from build123d import *

# Parameters (mm, degrees)
F1_DEPTH = 1
F3_D     = 8.64
F4_DEPTH = 25


with BuildPart() as f1:
    # F0 (on Top) → F1 (new body)
    with BuildSketch(Plane.XY):
        with BuildLine():
            Line((-21.45, 0), (0, 0))
            Line((0, 0), (21.45, 0))
            Line((21.45, 0), (22.2075974907, 8.6593789428))
            ThreePointArc((22.2075974907, 8.6593789428), (26.2007214664, 23.5619205011), (35.05, 36.2))
            ThreePointArc((35.05, 36.2), (33.1464754087, 101.0395325209), (39.45, 165.6))
            ThreePointArc((39.45, 165.6), (33.5426879174, 164.8198684719), (27.5886514491, 165.0530872052))
            ThreePointArc((27.5886514491, 165.0530872052), (24.9545680687, 165.6778337109), (22.5167661948, 166.8550445988))
            ThreePointArc((22.5167661948, 166.8550445988), (13.834235102, 170.9953697151), (4.4430186473, 173.0771218005))
            ThreePointArc((4.4430186473, 173.0771218005), (1.3309419019, 172.0659808949), (0, 169.0766630372))
            ThreePointArc((0, 169.0766630372), (-1.3309419019, 172.0659808949), (-4.4430186473, 173.0771218005))
            ThreePointArc((-4.4430186473, 173.0771218005), (-13.834235102, 170.9953697151), (-22.5167661948, 166.8550445988))
            ThreePointArc((-22.5167661948, 166.8550445988), (-24.9545680687, 165.6778337109), (-27.5886514491, 165.0530872052))
            ThreePointArc((-27.5886514491, 165.0530872052), (-33.5426879174, 164.8198684719), (-39.45, 165.6))
            ThreePointArc((-39.45, 165.6), (-33.1464754087, 101.0395325209), (-35.05, 36.2))
            ThreePointArc((-35.05, 36.2), (-26.2007214664, 23.5619205011), (-22.2075974907, 8.6593789428))
            Line((-22.2075974907, 8.6593789428), (-21.45, 0))
        make_face()
    extrude(amount=F1_DEPTH)

    # F3 (through all)
    with Locations(Plane.XY.offset(1)):
        with Locations((-19.51, 57.48), (-21.1084226467, 92.68), (-22.7068452934, 127.88), (22.7068452934, 127.88), (21.1084226467, 92.68), (19.51, 57.48)):
            Hole(F3_D / 2)

    # F5 (on face) → F4 (cut)
    with BuildSketch(Plane.XY.offset(1)):
        with BuildLine():
            Line((-8, 14), (0, 14))
            Line((0, 14), (8, 14))
            Line((8, 14), (8, 36))
            add(Edge.make_bspline(
                [(8, 36), (8, 56), (0, 56), (-8, 56), (-8, 36)],
                knots=[4.7123889804, 4.7123889804, 4.7123889804, 6.2831853072, 6.2831853072, 7.853981634, 7.853981634, 7.853981634], degree=2, weights=[1, 0.7071067812, 1, 0.7071067812, 1]))
            Line((-8, 36), (-8, 14))
        make_face()
    extrude(amount=-F4_DEPTH, mode=Mode.SUBTRACT)


solid = f1.part
Work out the finished part from the listing and answer in its coordinate system (mm). Round coordinates to 2 decimals unless told otherwise and drop trailing zeros. Write each loop counter-clockwise with the first axis right and the second up, starting at its lowest first coordinate (ties: lowest second). Pieces come first, ordered by that corner, then holes.
1) A cutting plane is placed at B-B (y = 17.5). Give the vertices of the cut face in (x, z).
2) A cutting plane is placed at D-D (y = 92.68). Give the vertices of the cut face in (x, z), plus the area to 3 significant figures.
3) A cutting plane is placed at A-A (y = 127.88). Give the vertices of the cut face in (x, z), plus the area to 4 significant figures.
4) A cutting plane is placed at C-C (z = 0.5). Give the number of separate pieces and of enclosed holes in the cut face, plus the area to 3 significant figures.
5) Straight lines are drawn through the part: line 1 (Y direction, x = -18, z = 0.2); line 2 (Y direction, x = 19.51, z = 0.65); line 3 (Y direction, x = 20, z = 0.95). For each, find the intervals that lie inside material, in ascending order.
Completed:
1. outline: (-23.9, 0) - (-8, 0) - (-8, 1) - (-23.9, 1) - close; (8, 0) - (23.9, 0) - (23.9, 1) - (8, 1) - close
2. outline: (-32.93, 0) - (-25.43, 0) - (-25.43, 1) - (-32.93, 1) - close; (-16.79, 0) - (16.79, 0) - (16.79, 1) - (-16.79, 1) - close; (25.43, 0) - (32.93, 0) - (32.93, 1) - (25.43, 1) - close
2. area: 48.6 mm2
3. outline: (-34.77, 0) - (-27.03, 0) - (-27.03, 1) - (-34.77, 1) - close; (-18.39, 0) - (18.39, 0) - (18.39, 1) - (-18.39, 1) - close; (27.03, 0) - (34.77, 0) - (34.77, 1) - (27.03, 1) - close
3. area: 52.25 mm2
4. separate pieces: 1
4. enclosed holes: 7
4. area: 10,100 mm2
5. line 1: y = 0 to 53.43, 61.53 to 89.68, 95.68 to 169.31
5. line 2: y = 0 to 53.16, 61.8 to 88.67, 96.69 to 124.97, 130.79 to 168.57
5. line 3: y = 0 to 53.19, 61.77 to 88.5, 96.86 to 124.51, 131.25 to 168.31
